from build123d import *

# Parameters (mm, degrees)
SKETCH_1_W          = 55
SKETCH_1_H          = 25
EXTRUDE_1_DEPTH     = 1.5
CUT_EXTRUDE_1_DEPTH = 61.433848132
SKETCH_3_R          = 1.6
CUT_EXTRUDE_2_DEPTH = 61.433848132


with BuildPart() as part:
    # Эскиз1 → Бобышка-Вытянуть1 (new body)
    with BuildSketch(Plane.XY):
        with Locations((27.5, 12.5)):
            Rectangle(SKETCH_1_W, SKETCH_1_H)
    extrude(amount=EXTRUDE_1_DEPTH)

    # Эскиз2 → Вырез-Вытянуть1 (cut, through all)
    with BuildSketch(Plane.XY.offset(1.5)):
        with BuildLine():
            Line((2, 18.75), (5, 18.75))
            ThreePointArc((5, 18.75), (6.6, 17.15), (5, 15.55))
            Line((5, 15.55), (2, 15.55))
            ThreePointArc((2, 15.55), (0.4, 17.15), (2, 18.75))
        make_face()
        with BuildLine():
            Line((53, 18.75), (50, 18.75))
            ThreePointArc((50, 18.75), (48.4, 17.15), (50, 15.55))
            Line((50, 15.55), (53, 15.55))
            ThreePointArc((53, 15.55), (54.6, 17.15), (53, 18.75))
        make_face()
    extrude(amount=-CUT_EXTRUDE_1_DEPTH, mode=Mode.SUBTRACT)

    # Эскиз3 → Вырез-Вытянуть2 (cut, through all)
    with BuildSketch(Plane.XY.offset(1.5)):
        with Locations((27.5, 22)):
            Circle(SKETCH_3_R)
        with Locations((27.5, 3)):
            Circle(SKETCH_3_R)
    extrude(amount=-CUT_EXTRUDE_2_DEPTH, mode=Mode.SUBTRACT)


solid = part.part
For this review, take the finished solid that the model builds, in its own axes (mm). A direction names the side the tool comes from. Round coordinates to 2 decimals unless told otherwise and drop trailing zeros. Loops run counter-clockwise (first coordinate to the right, second up) from the corner with the lowest first, then second, coordinate; pieces in that order, holes last. Notation, with made-up numbers: (51.25, 23.5) - (89.25, 23.5) arc R32 ccw to (89.25, 62.5) - close; hole circle Ø2 at (-7.75, 11). An arc over 180 degrees is marked (long way). Put each result on its own line as item: value. Start each with the question number.
1. For faces 1 (the flat face through (27, 13, 0)), 2 (the flat face through (52, 18.75, 1)), list the 3-axis set-ups (+Z, -Z, +X, -X, +Y, -Y) from which the entire face can be reached by the end or side of a thin tool; tool diameter is ignored.
2. For probe 1 along Y at (x, z) = (27.5, 0.95); probe 2 along Y at (x, z) = (27, 0.3); probe 3 along Y at (x, z) = (4, 1.2), list the stretches that pass through material, from the lowest coordinate up. Write a range as [from, to].
3. Consider section D-D on z = 0.45. State the section outline as (x, y) points, plus the area to 3 significant figures.
4. Consider section B-B on x = 27.5. State the section outline as (y, z) points.
5. Insertion check: P1, Ø1.9, axis at x = 27.5, y = 3, coming from the +Z side. The pin has a flat end and moves straight along its axis. Give the tip position at first contact, or say it passes through.
6. Consider section A-A on y = 17.15. State the section outline as (x, z) points, plus the area to 3 significant figures.
7. Consider section C-C on y = 22. State the section outline as (x, z) points, plus the area to 3 significant figures.
Result sheet:
1. face 1: -Z, +X, -X, +Y, -Y
1. face 2: +Z, -Z
2. probe 1: [0, 1.4], [4.6, 20.4], [23.6, 25]
2. probe 2: [0, 1.48], [4.52, 20.48], [23.52, 25]
2. probe 3: [0, 15.55], [18.75, 25]
3. outline: (0, 0) - (55, 0) - (55, 25) - (0, 25) - close; hole (2, 15.55) - (5, 15.55) arc R1.6 ccw to (5, 18.75) - (2, 18.75) arc R1.6 ccw to start; hole circle Ø3.2 at (27.5, 3); hole circle Ø3.2 at (27.5, 22); hole (50, 15.55) - (53, 15.55) arc R1.6 ccw to (53, 18.75) - (50, 18.75) arc R1.6 ccw to start
3. area: 1,320 mm^2
4. outline: (0, 0) - (1.4, 0) - (1.4, 1.5) - (0, 1.5) - close; (4.6, 0) - (20.4, 0) - (20.4, 1.5) - (4.6, 1.5) - close; (23.6, 0) - (25, 0) - (25, 1.5) - (23.6, 1.5) - close
5. P1: through
6. outline: (0, 0) - (0.4, 0) - (0.4, 1.5) - (0, 1.5) - close; (6.6, 0) - (48.4, 0) - (48.4, 1.5) - (6.6, 1.5) - close; (54.6, 0) - (55, 0) - (55, 1.5) - (54.6, 1.5) - close
6. area: 63.9 mm^2
7. outline: (0, 0) - (25.9, 0) - (25.9, 1.5) - (0, 1.5) - close; (29.1, 0) - (55, 0) - (55, 1.5) - (29.1, 1.5) - close
7. area: 77.7 mm^2
